Check sheet for the modelled part. Datum: model origin and axes. Units: mm. A direction names the side the tool comes from. Round coordinates to 2 decimals unless told otherwise and drop trailing zeros. Order: outer loops, then holes, each group sorted by start corner. A loop starts at its lowest first (then second) coordinate and runs counter-clockwise, first axis right, second up.
(1) Sectioned sample at C-C, the plane x = -52.75. Enter the section's corners in (y, z), and give its area (3 significant figures).
(2) Mould release check, pull along X, two halves, no side actions. Record for faces 1 (the cylindrical face through (-58.665, -1.252, 44.626)), 2 (the flat face through (-33.423, -1.252, 34.312)), 3 (the flat face through (-39, 0, 10)), 4 (the cylindrical face through (-43.805, -1.288, 23.455)): released by +X, released by -X, zero draft, split by the parting line, or undercut.
(3) Sectioned sample at A-A, the plane z = -7. Enter the section's corners in (x, y) (3 decimals).
(4) Depth check by flat-ended pin: pin 1 (1.3 mm diameter, centred on y = -2, z = 41, fed in from +X); pin 2 (1.5 mm diameter, centred on x = -37.5, y = -2, fed in from +Z); pin 3 (1.5 mm diameter, centred on y = -0.5, z = -12, fed in from -X). Enter the tip coordinate at first touch or a pass-through.
(5) Sectioned sample at B-B, the plane y = -1.35. Enter the section's corners in (x, z) (3 decimals).
(6) Tool access check on faces 5 (the flat face through (-49.938, -1, -8)), 6 (the flat face through (-49.938, -1, 40)), 7 (the flat face through (-37.238, -1, -9)), 8 (the cylindrical face through (-28.94, -1.25, 44.48)), 9 (the flat face through (-47.776, -1, -10)). Record the directions out of +Z, -Z, +X, -X, +Y, -Y that give a thin tool (end or side, any length) a straight path to the whole face; none if there is none.
(7) Sectioned sample at D-D, the plane z = 30.5. Enter the section's corners in (x, y), and give its area (3 significant figures).
(8) Thickness scan on probe 1 along X at (y, z) = (-0.9, 6) (3 decimals); probe 2 along Z at (x, y) = (-44.25, -1); probe 3 along Z at (x, y) = (-45.5, -1.35). Record the ranges inside material, lowest first.
```python
from build123d import *

# Parameters (mm, degrees)
F1_DEPTH    = 2.54
F2_T1_DEPTH = 21.3951912934
F2_T3_DEPTH = 22.4631654102
F2_T5_DEPTH = 27.94
F2_T7_DEPTH = 60.9088837652
F2_T9_DEPTH = 60.1042195061
F4_DEPTH    = 2.541


# Not quite as in the source:
# - a fillet or chamfer that OpenCascade refuses, or shapes differently, is made with other operations: its cross-section is extruded or revolved along the edge and cut away or added


with BuildPart() as f1:
    # F0 (on Front) → F1 (new body)
    with BuildSketch(Plane.XZ):
        Polygon((-49.9376785943, 26.895446232), (-49.9376785943, -49.304553768), (-37.2376785943, -49.304553768), (-37.2376785943, 26.895446232), (-27.7746748179, 45.2916584909), (-37.2376785943, 54.4446781278), (-37.5589355826, 37.401124835), (-49.9376785943, 37.401124835), (-49.9376785943, 54.4446781278), (-59.968046844, 45.2916584909), align=None)
    extrude(amount=F1_DEPTH)

    # F2: fillet of radius 5.08 on 6 edges, made by hand

    # F2_s2 → F2_t1 (cut)
    with BuildSketch(Plane.XZ.offset(-9.4275956467)):
        with BuildLine():
            ThreePointArc((-29.49965362, 41.9382754706), (-29.0047534445, 45.0887624488), (-30.4852273769, 47.9134201836))
            Line((-30.4852273769, 47.9134201836), (-27.7746748179, 45.2916584909))
            Line((-27.7746748179, 45.2916584909), (-29.49965362, 41.9382754706))
        make_face()
    extrude(amount=F2_T1_DEPTH, mode=Mode.SUBTRACT)

    # F2_s4 → F2_t3 (cut)
    with BuildSketch(Plane.XZ.offset(-9.9615827051)):
        with BuildLine():
            ThreePointArc((-57.0247017985, 47.9775514042), (-58.6106651129, 45.064296855), (-58.0605727295, 41.7932526681))
            Line((-58.0605727295, 41.7932526681), (-59.968046844, 45.2916584909))
            Line((-59.968046844, 45.2916584909), (-57.0247017985, 47.9775514042))
        make_face()
    extrude(amount=F2_T3_DEPTH, mode=Mode.SUBTRACT)

    # F2_s6 → F2_t5 (cut)
    with BuildSketch(Plane.XZ.offset(-12.7)):
        with BuildLine():
            ThreePointArc((-42.3176785943, -49.304553768), (-38.7255761459, -47.8166562165), (-37.2376785943, -44.224553768))
            Line((-37.2376785943, -44.224553768), (-37.2376785943, -49.304553768))
            Line((-37.2376785943, -49.304553768), (-42.3176785943, -49.304553768))
        make_face()
        with BuildLine():
            ThreePointArc((-49.9376785943, -44.224553768), (-48.4497810427, -47.8166562165), (-44.8576785943, -49.304553768))
            Line((-44.8576785943, -49.304553768), (-49.9376785943, -49.304553768))
            Line((-49.9376785943, -49.304553768), (-49.9376785943, -44.224553768))
        make_face()
    extrude(amount=F2_T5_DEPTH, mode=Mode.SUBTRACT)

    # F2_s8 → F2_t7 (cut)
    with BuildSketch(Plane.XZ.offset(-29.1844418826)):
        with BuildLine():
            ThreePointArc((-28.8467837584, 46.3286478461), (-34.3174578503, 47.3726785237), (-37.457680624, 42.7729746194))
            Line((-37.457680624, 42.7729746194), (-37.2376785943, 54.4446781278))
            Line((-37.2376785943, 54.4446781278), (-28.8467837584, 46.3286478461))
        make_face()
    extrude(amount=F2_T7_DEPTH, mode=Mode.SUBTRACT)

    # F2_s10 → F2_t9 (cut)
    with BuildSketch(Plane.XZ.offset(-28.782109753)):
        with BuildLine():
            ThreePointArc((-49.9376785943, 42.9318342266), (-52.9669146048, 47.5794967637), (-58.4419175941, 46.6842983866))
            Line((-58.4419175941, 46.6842983866), (-49.9376785943, 54.4446781278))
            Line((-49.9376785943, 54.4446781278), (-49.9376785943, 42.9318342266))
        make_face()
    extrude(amount=F2_T9_DEPTH, mode=Mode.SUBTRACT)

    # F3 (on face) → F4 (cut, through all)
    with BuildSketch(Plane.XZ.offset(2.54)):
        with BuildLine():
            Line((-40.0050021708, -40.580611676), (-40.0050021708, 19.5707920939))
            ThreePointArc((-40.0050021708, 19.5707920939), (-43.8903793693, 23.4561692923), (-47.7757565677, 19.5707920939))
            Line((-47.7757565677, 19.5707920939), (-47.7757565677, -40.580611676))
            ThreePointArc((-47.7757565677, -40.580611676), (-43.8903793693, -44.4659888744), (-40.0050021708, -40.580611676))
        make_face()
    extrude(amount=-F4_DEPTH, mode=Mode.SUBTRACT)


solid = f1.part
```
Derived:
1. outline: (-2.54, 32.05) - (0, 32.05) - (0, 47.48) - (-2.54, 47.48) - close
1. area: 39.2 mm2
2. face 1: released by -X
2. face 2: released by +X
2. face 3: zero draft
2. face 4: undercut
3. outline: (-49.938, -2.54) - (-47.776, -2.54) - (-47.776, 0) - (-49.938, 0) - close; (-40.005, -2.54) - (-37.238, -2.54) - (-37.238, 0) - (-40.005, 0) - close
4. pin 1: stops at x = -29.65
4. pin 2: stops at z = 45.27
4. pin 3: stops at x = -49.94
5. outline: (-58.061, 41.793) - (-49.938, 26.895) - (-49.938, -44.225) arc R5.08 ccw to (-44.858, -49.305) - (-42.318, -49.305) arc R5.08 ccw to (-37.238, -44.225) - (-37.238, 26.895) - (-29.5, 41.938) arc R5.08 ccw to (-29.756, 47.028) arc R5.08 ccw to (-37.458, 42.773) - (-37.559, 37.401) - (-49.938, 37.401) - (-49.938, 42.932) arc R5.08 ccw to (-57.672, 47.263) arc R5.08 ccw to start; hole (-47.776, -40.581) arc R3.885 ccw to (-40.005, -40.581) - (-40.005, 19.571) arc R3.885 ccw to (-47.776, 19.571) - close
6. face 5: -Z, -X, +Y, -Y
6. face 6: +Z, +Y, -Y
6. face 7: -Z, +X, +Y, -Y
6. face 8: +X, +Y, -Y
6. face 9: +Y, -Y
7. outline: (-51.9, -2.54) - (-35.38, -2.54) - (-35.38, 0) - (-51.9, 0) - close
7. area: 42.0 mm2
8. probe 1: x = -49.938 to -47.776, -40.005 to -37.238
8. probe 2: z = -49.3 to -44.45, 23.44 to 37.4
8. probe 3: z = -49.26 to -44.12, 23.11 to 37.4
